from build123d import *

# Parameters (mm, degrees)
BODY_START                       = 1.25
BODY_DEPTH                       = 11.75
PEG_DEPTH                        = 6
CHAMFER1_SIZE                    = 0.5
M2_5_CLEARANCE_HOLE1_D           = 2.7
M2_5_CLEARANCE_HOLE1_CSINK_D     = 2.75
M2_5_CLEARANCE_HOLE1_CSINK_ANGLE = 90
FILLET3_R                        = 0.75


with BuildPart() as part:
    # Sketch2 → body (new body)
    with BuildSketch(Plane.ZY.offset(29.5).offset(BODY_START)):
        with BuildLine():
            Line((2.75, -3), (0, -3))
            Line((0, -3), (0, 3))
            Line((0, 3), (2.75, 3))
            ThreePointArc((2.75, 3), (5.75, 0), (2.75, -3))
        make_face()
    extrude(amount=BODY_DEPTH)

    # Sketch3 → peg (add)
    with BuildSketch(Plane(origin=(0, 0, 0), x_dir=(-1, 0, 0), z_dir=(0, 0, -1))):
        with BuildLine():
            Line((35.1, 1.4), (39.9, 1.4))
            ThreePointArc((39.9, 1.4), (40.607106781, 1.107106781), (40.9, 0.4))
            Line((40.9, 0.4), (40.9, -0.4))
            ThreePointArc((40.9, -0.4), (40.607106781, -1.107106781), (39.9, -1.4))
            Line((39.9, -1.4), (35.1, -1.4))
            ThreePointArc((35.1, -1.4), (34.392893219, -1.107106781), (34.1, -0.4))
            Line((34.1, -0.4), (34.1, 0.4))
            ThreePointArc((34.1, 0.4), (34.392893219, 1.107106781), (35.1, 1.4))
        make_face()
    extrude(amount=PEG_DEPTH)

    # Chamfer1
    chamfer1_edges = [part.edges().sort_by_distance(p)[0] for p in [
        (-34.392893219, 1.107106781, -6),
        (-34.1, 0, -6),
        (-34.392893219, -1.107106781, -6),
        (-37.5, -1.4, -6),
        (-40.607106781, -1.107106781, -6),
        (-40.9, 0, -6),
        (-40.607106781, 1.107106781, -6),
        (-37.5, 1.4, -6),
    ]]
    chamfer(chamfer1_edges, length=CHAMFER1_SIZE)

    # Sketch5 → 9/64 (0.14063) Diameter Hole1 (revolve, cut)
    with BuildSketch(Plane(origin=(-30.75, 0, 2.75), x_dir=(0, 0, -1), z_dir=(0, 1, 0))):
        Polygon((0, 0), (0, 8.073137666), (1.786001, 7), (1.786001, 3.881186521), (2.0574, 0), align=None)
    revolve(axis=Axis((-24.4, 0, 2.75), (-1, 0, 0)), mode=Mode.SUBTRACT)

    # M2.5 Clearance Hole1 (through all)
    with Locations(Plane.ZY.offset(42.5)):
        with Locations((2.75, 0)):
            CounterSinkHole(M2_5_CLEARANCE_HOLE1_D / 2, M2_5_CLEARANCE_HOLE1_CSINK_D / 2, counter_sink_angle=M2_5_CLEARANCE_HOLE1_CSINK_ANGLE)

    # Fillet3
    fillet3_edges = [part.edges().sort_by_distance(p)[0] for p in [
        (-42.5, -3, 1.375),
        (-42.5, 0, 5.75),
        (-30.75, -3, 1.375),
        (-30.75, 3, 1.375),
        (-30.75, 0, 5.75),
        (-42.5, 3, 1.375),
    ]]
    fillet(fillet3_edges, radius=FILLET3_R)


solid = part.part
CAD build for the part. Positions are in the model's coordinates, mm. A direction names the side the tool comes from. Round coordinates to 2 decimals unless told otherwise and drop trailing zeros. Loops run counter-clockwise (first coordinate to the right, second up) from the corner with the lowest first, then second, coordinate; pieces in that order, holes last. Notation, with made-up numbers: M 31.5,18.5 L 49.5,18.5 A17 cw 49.5,39.5 Z; hole C 4.5,86 d3. An arc over 180 degrees is marked long. One line per question, with ' | ' between items. Start each with the question number.
Item 1: Two-plate mould, pull along Z, no slides. Class faces 4 (the cylindrical face through (-34.385, 1.099, -2.712)), 5 (the cylindrical face through (-36.169, -1.207, 4.066)), 6 (the flat face through (-37, -2, 0)): pulls with the +Z half, pulls with the -Z half, needs draft (parallel to the pull), parting line crosses it, or undercut.
Item 2: Which spindle directions (+Z, -Z, +X, -X, +Y, -Y) get a long thin tool onto all of the face, cutting with end or side? Do faces 1 (the cylindrical face through (-40.615, -1.099, -2.712)), 2 (the cylindrical face through (-34.401, -1.115, -2.712)), 3 (the cylindrical face through (-40.599, 1.115, -2.712)). Say none if no direction does.
Item 3: Cut at C-C, the plane z = -4. Write the cut outline in (x, y).
Item 4: Pin check, flat tips, straight feed: pin 1 Ø6 at (x, z) = (-35.5, -4) entering from -Y; pin 2 Ø1 at (y, z) = (-0.5, 2.5) entering from +X; pin 3 Ø3 at (y, z) = (1.5, -4) entering from -X; pin 4 Ø5.5 at (x, z) = (-38.5, -3) entering from +Y. Stop position of each tip, or through.
Item 5: Cut at A-A, the plane x = -35.5. Write the cut outline in (y, z), plus the area to 3 significant figures.
Item 6: Wall check: line 1 (Z direction, x = -36.1, y = 0); line 2 (Z direction, x = -40.25, y = 0); line 3 (Y direction, x = -35.55, z = 2.75). Give the ranges that are in metal, low to high.
Item 7: Cut at B-B, the plane y = 0. Write the cut outline in (x, z) (3 decimals).
Item 8: Cut at D-D, the plane x = -39. Write the cut outline in (y, z), plus the area to 3 significant figures.
Responses:
1) face 4: needs draft | face 5: undercut | face 6: pulls with the -Z half
2) face 1: -Z, -X, -Y | face 2: -Z, +X, -Y | face 3: -Z, -X, +Y
3) outline: M -40.9,-0.4 A1 ccw -39.9,-1.4 L -35.1,-1.4 A1 ccw -34.1,-0.4 L -34.1,0.4 A1 ccw -35.1,1.4 L -39.9,1.4 A1 ccw -40.9,0.4 Z
4) pin 1: stops at y = -1.4 | pin 2: passes through | pin 3: stops at x = -40.9 | pin 4: stops at y = 1.4
5) outline: M -3,0 L -1.4,0 L -1.4,-5.5 L -0.9,-6 L 0.9,-6 L 1.4,-5.5 L 1.4,0 L 3,0 L 3,2.75 A3 ccw -3,2.75 Z; hole C 0,2.75 d3.57 | area: 37.2 mm²
6) line 1: z = -6 to 0.96, 4.54 to 5.75 | line 2: z = -6 to 1.4, 4.1 to 5.75 | line 3: y = -3 to -1.79, 1.79 to 3
7) outline: M -42.5,0 L -40.9,0 L -40.9,-5.5 L -40.4,-6 L -34.6,-6 L -34.1,-5.5 L -34.1,0 L -30.75,0 L -30.75,0.693 L -34.631,0.964 L -37.75,0.964 L -38.012,1.4 L -42.475,1.4 L -42.5,1.375 Z; M -42.5,4.125 L -42.475,4.1 L -38.012,4.1 L -37.75,4.536 L -34.631,4.536 L -30.75,4.807 L -30.75,5 A0.75 ccw -31.5,5.75 L -41.75,5.75 A0.75 ccw -42.5,5 Z
8) outline: M -3,0 L -1.4,0 L -1.4,-5.5 L -0.9,-6 L 0.9,-6 L 1.4,-5.5 L 1.4,0 L 3,0 L 3,2.75 A3 ccw -3,2.75 Z; hole C 0,2.75 d2.7 | area: 41.5 mm²
